Input: part model. Units: mm. Frame: model coordinates. A direction names the side the tool comes from. Give positions to 0.01 mm unless a question says otherwise; leave off trailing zeros. Loops run counter-clockwise (first coordinate to the right, second up) from the corner with the lowest first, then second, coordinate; pieces in that order, holes last. Notation, with made-up numbers: (-8, 68.5) -> (1, 68.5) arc R23 cw to (1, 79.5) -> close; hole circle Ø7 at (-27.75, -25). An arc over 180 degrees is marked (long way). Use CSV: the item, a comma, the result in double quotes.
```python
from build123d import *

# Parameters (mm, degrees)
SKETCH1_W           = 75
SKETCH1_H           = 67
SKETCH1_W_2         = 65
SKETCH1_H_2         = 57
BOSS_EXTRUDE1_DEPTH = 1.6
SKETCH2_W           = 5
SKETCH2_H           = 16.553638176
BOSS_EXTRUDE2_DEPTH = 5.5
SKETCH3_W           = 2.5
SKETCH3_H           = 67
BOSS_EXTRUDE3_DEPTH = 6
CUT_EXTRUDE1_REACH  = 102.747
CUT_EXTRUDE2_REACH  = 102.747
CUT_EXTRUDE3_REACH  = 102.747


with BuildPart() as part:
    # Sketch1 → Boss-Extrude1 (new body)
    with BuildSketch(Plane(origin=(0, 0, 0), x_dir=(1, 0, 0), z_dir=(0, 1, 0))):
        with Locations((37.5, 33.5)):
            Rectangle(SKETCH1_W, SKETCH1_H)
        with Locations((37.5, 33.5)):
            Rectangle(SKETCH1_W_2, SKETCH1_H_2, mode=Mode.SUBTRACT)
    extrude(amount=BOSS_EXTRUDE1_DEPTH)

    # Sketch2 → Boss-Extrude2 (add)
    with BuildSketch(Plane(origin=(0, 0, 0), x_dir=(-1, 0, 0), z_dir=(0, -1, 0))):
        with Locations((-72.5, 8.276819088)):
            Rectangle(SKETCH2_W, SKETCH2_H)
    extrude(amount=BOSS_EXTRUDE2_DEPTH)

    # Sketch3 → Boss-Extrude3 (add)
    with BuildSketch(Plane(origin=(0, 0, 0), x_dir=(-1, 0, 0), z_dir=(0, -1, 0))):
        with Locations((-1.25, 33.5)):
            Rectangle(SKETCH3_W, SKETCH3_H)
    extrude(amount=BOSS_EXTRUDE3_DEPTH)

    # Sketch4 → Cut-Extrude1 (cut, up to next)
    with BuildSketch(Plane.XY, mode=Mode.PRIVATE) as cut_extrude1_sk1:
        with BuildLine():
            Line((2.5, -3.843145751), (2.5, -6))
            Line((2.5, -6), (1.208438024, -6))
            ThreePointArc((1.208438024, -6), (1.778538223, -4.876253897), (2.5, -3.843145751))
        make_face()
    cut_extrude1_tool1 = extrude(cut_extrude1_sk1.sketch, amount=-CUT_EXTRUDE1_REACH, mode=Mode.PRIVATE) & part.part
    add(cut_extrude1_tool1.solids().sort_by_distance((2.045896, -5.244781, 0))[0], mode=Mode.SUBTRACT)

    # Sketch5 → Cut-Extrude2 (cut, up to next)
    with BuildSketch(Plane.ZY, mode=Mode.PRIVATE) as cut_extrude2_sk1:
        with BuildLine():
            Line((-12, -6), (-55, -6))
            add(Edge.make_bspline(
                [(-55, -6), (-33.5, 4), (-12, -6)],
                knots=[0, 0, 0, 1, 1, 1], degree=2))
        make_face()
    cut_extrude2_tool1 = extrude(cut_extrude2_sk1.sketch, amount=-CUT_EXTRUDE2_REACH, mode=Mode.PRIVATE) & part.part
    add(cut_extrude2_tool1.solids().sort_by_distance((0, -4, -33.5))[0], mode=Mode.SUBTRACT)

    # Sketch6 → Cut-Extrude3 (cut, up to next)
    with BuildSketch(Plane(origin=(75, 0, 0), x_dir=(0, 0, -1), z_dir=(1, 0, 0)), mode=Mode.PRIVATE) as cut_extrude3_sk1:
        with BuildLine():
            Line((16.553638176, -1.377553515), (16.553638176, -5.5))
            Line((16.553638176, -5.5), (10.16876266, -5.5))
            ThreePointArc((10.16876266, -5.5), (13.054139073, -2.963197882), (16.553638176, -1.377553515))
        make_face()
    cut_extrude3_tool1 = extrude(cut_extrude3_sk1.sketch, amount=-CUT_EXTRUDE3_REACH, mode=Mode.PRIVATE) & part.part
    # Sketch6 → Cut-Extrude3 (cut, up to next)
    with BuildSketch(Plane(origin=(75, 0, 0), x_dir=(0, 0, -1), z_dir=(1, 0, 0)), mode=Mode.PRIVATE) as cut_extrude3_sk2:
        with BuildLine():
            Line((4.215785495, -5.5), (0, -5.5))
            Line((0, -5.5), (0, -0.880945509))
            ThreePointArc((0, -0.880945509), (2.338832837, -2.979695012), (4.215785495, -5.5))
        make_face()
    cut_extrude3_tool2 = extrude(cut_extrude3_sk2.sketch, amount=-CUT_EXTRUDE3_REACH, mode=Mode.PRIVATE) & part.part
    add(cut_extrude3_tool1.solids().sort_by_distance((75, -3.96823, -14.212135))[0], mode=Mode.SUBTRACT)
    add(cut_extrude3_tool2.solids().sort_by_distance((75, -3.859275, -1.499307))[0], mode=Mode.SUBTRACT)


solid = part.part
```
1) Section query C-C (z = -58). Return loops of the section in (x, y), then the cut area to 3 significant figures.
From the geometry:
outline,"(0, -6) -> (1.21, -6) arc R9 cw to (2.5, -3.84) -> (2.5, 0) -> (5, 0) -> (5, 1.6) -> (0, 1.6) -> close; (70, 0) -> (75, 0) -> (75, 1.6) -> (70, 1.6) -> close"
area,"29.5 mm^2"
2) Ray query, line 1 (Z direction, x = 6.5, y = 1); line 2 (X direction, y = 1.25, z = -56.5); line 3 (X direction, y = -0.25, z = -8). Return the intervals inside material, ascending.
From the geometry:
line 1,"z = -67 to -62, -5 to 0"
line 2,"x = 0 to 5, 70 to 75"
line 3,"x = 0 to 2.5, 70 to 75"
3) Section query A-A (z = -6.5). Return loops of the section in (x, y), then the cut area to 3 significant figures.
From the geometry:
outline,"(0, -6) -> (1.21, -6) arc R9 cw to (2.5, -3.84) -> (2.5, 0) -> (5, 0) -> (5, 1.6) -> (0, 1.6) -> close; (70, -5.5) -> (75, -5.5) -> (75, 1.6) -> (70, 1.6) -> close"
area,"57.0 mm^2"
4) Reachability of faces 1 (the cylindrical face through (1.77, -4.89, -6.6)), 2 (the flat face through (37, 1, -62)), 3 (the cylindrical face through (73, -3, -13)) from +Z, -Z, +X, -X, +Y, -Y: full face, straight path, thin tool, end or side. Return the list, or none.
From the geometry:
face 1,"+Z, -Z, -Y"
face 2,"+Y, -Y"
face 3,"-Z, +X, -Y"
5) Mould query, pull axis Z, two halves, no side actions, for faces 4 (the flat face through (37, 1, -5)), 5 (the flat face through (41, 0, -63)), 6 (the cylindrical face through (72.54, -2.95, -2.31)). Classes: pulls with the +Z half, pulls with the -Z half, needs draft (parallel to the pull), parting line crosses it, or undercut.
From the geometry:
face 4,"undercut"
face 5,"needs draft"
face 6,"pulls with the +Z half"
6) Contact query for flat-ended pins moving along their axis: pin 1 (5.5 mm diameter, centred on x = 71.5, z = -8.5, fed in from -Y); pin 2 (1.9 mm diameter, centred on y = -1.5, z = -20, fed in from +X). Output: stop coordinate, or through.
From the geometry:
pin 1,"stops at y = -5.5"
pin 2,"stops at x = 2.5"
7) Section query B-B (x = 31.5). Return loops of the section in (y, z).
From the geometry:
outline,"(0, -67) -> (1.6, -67) -> (1.6, -62) -> (0, -62) -> close; (0, -5) -> (1.6, -5) -> (1.6, 0) -> (0, 0) -> close"
